For this review, take the finished solid that the model builds, in its own axes (mm). Round coordinates to 2 decimals unless told otherwise and drop trailing zeros. Loops run counter-clockwise (first coordinate to the right, second up) from the corner with the lowest first, then second, coordinate; pieces in that order, holes last.
1. Consider section B-B on z = -6. State the section outline as (x, y) points.
2. Consider section A-A on y = 0. State the section outline as (x, z) points, then the cut area to 3 significant figures.
3. To check wall thickness, follow line 1 along Z through (x, y) = (-18, 0.05); line 2 along Z through (x, y) = (9, -0.5). State the ranges of each line that lie inside material, in increasing order.
4. Consider section C-C on x = 2.5. State the section outline as (y, z) points.
Autodesk Inventor part; units mm, degrees
ref_plane "YZ Plane" through (0, 0, 0) normal (1, 0, 0) x (0, 1, 0)
ref_plane "XZ Plane" through (0, 0, 0) normal (0, 1, 0) x (-1, 0, 0)
ref_plane "XY Plane" through (0, 0, 0) normal (0, 0, 1) x (1, 0, 0)
sketch "Sketch1" plane through (0, 0, 0) normal (0, 1, 0) x (-1, 0, 0)
  line L0 (-19.5, 22.5) -> (20.5, 22.5)
  line L1 (22.5, 20.5) -> (22.5, -19.5)
  line L2 (19.5, -22.5) -> (-19.5, -22.5)
  line L3 (-22.5, -19.5) -> (-22.5, 19.5)
  line L4 (-22.5, 22.5) -> (22.5, -22.5) construction
  line L5 (22.5, 22.5) -> (-22.5, -22.5) construction
  arc A0 (22.5, 20.5) -> (20.5, 22.5) centre (20.5, 20.5) ccw
  arc A1 (19.5, -22.5) -> (22.5, -19.5) centre (19.5, -19.5) ccw
  arc A2 (-22.5, -19.5) -> (-19.5, -22.5) centre (-19.5, -19.5) ccw
  arc A3 (-19.5, 22.5) -> (-22.5, 19.5) centre (-19.5, 19.5) ccw
  point P0 (0, 0)
  dimension "d0" = 45
  dimension "d1" = 45
  dimension "d2" = 2
  dimension "d3" = 3
sketch "Sketch2" plane through (0, 0, 0) normal (0, 0, 1) x (1, 0, 0)
  point P0 (0, 0)
sketch "Sketch3" plane through (0, 0, 0) normal (0, 0, 1) x (1, 0, 0)
  circle A0 centre (22.5, 0) radius 0.9712
  point P0 (0, 0)
  dimension "d5" = 22.5
sweep "Sweep1" add profiles "Sketch3" path "Sketch1"
equation "\"d1\" = d0"
properties part number "rfCoilSmaller"
Resolved:
1. outline: circle Ø1.94 at (-22.5, 0); circle Ø1.94 at (22.5, 0)
2. outline: (-23.47, -19.5) arc R3.97 ccw to (-19.5, -23.47) - (19.5, -23.47) arc R3.97 ccw to (23.47, -19.5) - (23.47, 19.5) arc R3.97 ccw to (19.5, 23.47) - (-20.5, 23.47) arc R2.97 ccw to (-23.47, 20.5) - close; hole (-21.53, -19.5) arc R2.03 ccw to (-19.5, -21.53) - (19.5, -21.53) arc R2.03 ccw to (21.53, -19.5) - (21.53, 19.5) arc R2.03 ccw to (19.5, 21.53) - (-20.5, 21.53) arc R1.03 ccw to (-21.53, 20.5) - close
2. area: 340 mm2
3. line 1: z = -23.47 to -21.53, 21.53 to 23.47
3. line 2: z = -23.33 to -21.67, 21.67 to 23.33
4. outline: circle Ø1.94 at (0, -22.5); circle Ø1.94 at (0, 22.5)
